from build123d import *

# Parameters (mm, degrees)
BOSS_EXTRUDE1_DEPTH     = 100
BOSS_EXTRUDE3_DEPTH     = 10
SKETCH4_R               = 1.5
CUT_EXTRUDE1_DEPTH      = 149
CUT_EXTRUDE1_DEPTH_BACK = 16
SKETCH5_R               = 1.5
CUT_EXTRUDE2_DEPTH      = 16
CUT_EXTRUDE2_DEPTH_BACK = 16
SKETCH6_R               = 1.5
CUT_EXTRUDE3_DEPTH      = 16
CUT_EXTRUDE3_DEPTH_BACK = 16
SKETCH7_R               = 1.5
CUT_EXTRUDE4_DEPTH      = 16
CUT_EXTRUDE4_DEPTH_BACK = 16


with BuildPart() as part:
    # Sketch1 → Boss-Extrude1 (new body)
    with BuildSketch(Plane.XY):
        with BuildLine():
            ThreePointArc((62.5, 0), (0, -62.5), (-62.5, 0))
            Line((-62.5, 0), (-67.5, 0))
            ThreePointArc((-67.5, 0), (0, -67.5), (67.5, 0))
            Line((67.5, 0), (62.5, 0))
        make_face()
    extrude(amount=BOSS_EXTRUDE1_DEPTH)

    # Sketch3 → Boss-Extrude3 (add)
    with BuildSketch(Plane.XY.offset(15)):
        with BuildLine():
            Line((-52.112697755, -24.30055005), (-56.64423669, -26.413641359))
            ThreePointArc((-56.64423669, -26.413641359), (-53.00300601, -33.119954015), (-48.571622591, -39.332524441))
            Line((-48.571622591, -39.332524441), (-44.685892784, -36.185922485))
            ThreePointArc((-44.685892784, -36.185922485), (-48.762765529, -30.470357693), (-52.112697755, -24.30055005))
        make_face()
        with BuildLine():
            Line((-7.007487246, -57.071403719), (-7.616833963, -62.034134478))
            ThreePointArc((-7.616833963, -62.034134478), (0, -62.5), (7.616833963, -62.034134478))
            Line((7.616833963, -62.034134478), (7.007487246, -57.071403719))
            ThreePointArc((7.007487246, -57.071403719), (0, -57.5), (-7.007487246, -57.071403719))
        make_face()
        with BuildLine():
            ThreePointArc((48.571622591, -39.332524441), (53.00300601, -33.119954015), (56.64423669, -26.413641359))
            Line((56.64423669, -26.413641359), (52.112697755, -24.30055005))
            ThreePointArc((52.112697755, -24.30055005), (48.762765529, -30.470357693), (44.685892784, -36.185922485))
            Line((44.685892784, -36.185922485), (48.571622591, -39.332524441))
        make_face()
    extrude(amount=BOSS_EXTRUDE3_DEPTH)

    # Sketch4 → Cut-Extrude1 (cut, two sides)
    with BuildSketch(Plane.ZY.offset(-62.5)) as cut_extrude1_sk:
        with Locations((6, -6)):
            Circle(SKETCH4_R)
    extrude(amount=CUT_EXTRUDE1_DEPTH, mode=Mode.SUBTRACT)
    extrude(cut_extrude1_sk.sketch, amount=-CUT_EXTRUDE1_DEPTH_BACK, mode=Mode.SUBTRACT)

    # Sketch5 → Cut-Extrude2 (cut, two sides)
    with BuildSketch(Plane(origin=(0, -62.5, 0), x_dir=(1, 0, 0), z_dir=(0, 1, 0))) as cut_extrude2_sk:
        with Locations((0, -6)):
            Circle(SKETCH5_R)
    extrude(amount=CUT_EXTRUDE2_DEPTH, mode=Mode.SUBTRACT)
    extrude(cut_extrude2_sk.sketch, amount=-CUT_EXTRUDE2_DEPTH_BACK, mode=Mode.SUBTRACT)

    # Sketch6 → Cut-Extrude3 (cut, two sides)
    with BuildSketch(Plane(origin=(-30.300601265, -54.663731696, 0), x_dir=(0.874619707, -0.48480962, 0), z_dir=(0.48480962, 0.874619707, 0))) as cut_extrude3_sk:
        with Locations((-0.663731696, -20)):
            Circle(SKETCH6_R)
    extrude(amount=CUT_EXTRUDE3_DEPTH, mode=Mode.SUBTRACT)
    extrude(cut_extrude3_sk.sketch, amount=-CUT_EXTRUDE3_DEPTH_BACK, mode=Mode.SUBTRACT)

    # Sketch7 → Cut-Extrude4 (cut, two sides)
    with BuildSketch(Plane(origin=(30.300601265, -54.663731696, 0), x_dir=(0.874619707, 0.48480962, 0), z_dir=(-0.48480962, 0.874619707, 0))) as cut_extrude4_sk:
        with Locations((0.663731696, -20)):
            Circle(SKETCH7_R)
    extrude(amount=CUT_EXTRUDE4_DEPTH, mode=Mode.SUBTRACT)
    extrude(cut_extrude4_sk.sketch, amount=-CUT_EXTRUDE4_DEPTH_BACK, mode=Mode.SUBTRACT)


solid = part.part
Input: part model. Units: mm. Frame: model coordinates. A direction names the side the tool comes from. Coordinates: 2 decimals unless noted, no trailing zeros. Order: outer loops, then holes, each group sorted by start corner. A loop starts at its lowest first (then second) coordinate and runs counter-clockwise, first axis right, second up. Notation, with made-up numbers: M 47,9.25 L 68,9.25 A15 ccw 68,29.25 Z; hole C 5.25,18.5 d6. An arc over 180 degrees is marked long. Answer in a Markdown table with one row per item.
(1) Material intervals for line 1 (Z direction, x = -64.6, y = -6); line 2 (X direction, y = -34, z = 45.5); line 3 (X direction, y = -55.5, z = 30), sorted ascending. Write a range as [from, to].
Numbers:
| item | result |
|---|---|
| line 1 | z = [0, 4.5], [7.5, 100] |
| line 2 | x = [-58.31, -52.44], [52.44, 58.31] |
| line 3 | x = [-38.42, -28.74], [28.74, 38.42] |
(2) Section query B-B, the plane x = 3. Output: boundary loops of the cut face in (y, z), plus the area to 3 significant figures.
Numbers:
| item | result |
|---|---|
| outline | M -67.43,0 L -62.43,0 L -62.43,15 L -57.42,15 L -57.42,25 L -62.43,25 L -62.43,100 L -67.43,100 Z |
| area | 551 mm^2 |
(3) Section query D-D, the plane x = 24. Output: boundary loops of the cut face in (y, z), plus the area to 3 significant figures.
Numbers:
| item | result |
|---|---|
| outline | M -63.09,0 L -57.71,0 L -57.71,100 L -63.09,100 Z |
| area | 538 mm^2 |
(4) Draft query along X for faces 1 (the flat face through (51, -32, 25)), 2 (the cylindrical face through (-1.484, -67.484, 49.3)), 3 (the flat face through (0, -60, 25)), 4 (the flat face through (65, 0, 49)). Return one class per face: pulls with the +X half, pulls with the -X half, needs draft (parallel to the pull), parting line crosses it, or undercut.
Numbers:
| item | result |
|---|---|
| face 1 | undercut |
| face 2 | parting line crosses it |
| face 3 | undercut |
| face 4 | needs draft |
(5) Section query C-C, the plane z = 37.5. Output: boundary loops of the cut face in (x, y), plus the area to 3 significant figures.
Numbers:
| item | result |
|---|---|
| outline | M -67.5,0 A67.5 ccw 67.5,0 L 62.5,0 A62.5 cw -62.5,0 Z |
| area | 1,020 mm^2 |
(6) Access query for faces 5 (the flat face through (0, -60, 15)), 6 (the flat face through (-7.31, -59.52, 19.93)), 7 (the flat face through (46.602, -37.737, 19.93)), 8 (the flat face through (0, -64, 0)). Directions: +Z, -Z, +X, -X, +Y, -Y. A direction counts if a zero-diameter tool reaches every point of the face in a straight line with its end or side. Return the directions, or none.
Numbers:
| item | result |
|---|---|
| face 5 | -Z, +Y |
| face 6 | +Z, -Z, +Y |
| face 7 | +Z, -Z |
| face 8 | -Z, +X, -X, +Y, -Y |
(7) Section query A-A, the plane y = -9.5. Output: boundary loops of the cut face in (x, z), plus the area to 3 significant figures.
Numbers:
| item | result |
|---|---|
| outline | M -66.83,0 L -61.77,0 L -61.77,100 L -66.83,100 Z; M 61.77,0 L 66.83,0 L 66.83,100 L 61.77,100 Z |
| area | 1,010 mm^2 |
(8) Contact query for flat-ended pins moving along their axis: pin 1 Ø3.5 at (x, y) = (47.5, -30) entering from -Z; pin 2 Ø5 at (x, z) = (40, 13.5) entering from +Y; pin 3 Ø6 at (y, z) = (-11.5, 75) entering from +X. Output: stop coordinate, or through.
Numbers:
| item | result |
|---|---|
| pin 1 | stops at z = 15 |
| pin 2 | stops at y = -45.83 |
| pin 3 | stops at x = 66.96 |
